Could you check a few things on this model? Use its own coordinates, in mm. Face numbers are marked on the shaded views. Round coordinates to 2 decimals unless told otherwise and drop trailing zeros. Order: outer loops, then holes, each group sorted by start corner. A loop starts at its lowest first (then second) coordinate and runs counter-clockwise, first axis right, second up.
```python
from build123d import *

# Parameters (mm, degrees)
EXTRUDE_1_DEPTH          = 30
SKETCH_2_R               = 3.5
CUT_EXTRUDE_1_DEPTH      = 71
SKETCH_3_R               = 3.5
CUT_EXTRUDE_2_DEPTH      = 71
SKETCH_4_R               = 4.5
SKETCH_4_R_2             = 2.5
EXTRUDE_2_DEPTH          = 30
SKETCH_5_R               = 2.5
CUT_EXTRUDE_6_DEPTH      = 31
SKETCH_6_W               = 11.97763243
SKETCH_6_H               = 9.98933257
CUT_EXTRUDE_8_DEPTH      = 71
CUT_EXTRUDE_8_DEPTH_BACK = 1.2


with BuildPart() as part:
    # Эскиз1 → Вытянуть-Тонкостенный1 (new body)
    with BuildSketch(Plane(origin=(0, 0, 0), x_dir=(1, 0, 0), z_dir=(0, 1, 0))):
        Polygon((0, 70), (0, 0), (70, 0), (70, 3), (3, 3), (3, 70), align=None)
    extrude(amount=EXTRUDE_1_DEPTH)

    # Эскиз2 → Вырез-Вытянуть1 (cut, through all)
    with BuildSketch(Plane.ZY):
        with Locations((-50, 20)):
            Circle(SKETCH_2_R)
        with Locations((-25, 10)):
            Circle(SKETCH_2_R)
    extrude(amount=-CUT_EXTRUDE_1_DEPTH, mode=Mode.SUBTRACT)

    # Эскиз3 → Вырез-Вытянуть2 (cut, through all)
    with BuildSketch(Plane.XY):
        with Locations((25, 20)):
            Circle(SKETCH_3_R)
        with Locations((50, 10)):
            Circle(SKETCH_3_R)
    extrude(amount=-CUT_EXTRUDE_2_DEPTH, mode=Mode.SUBTRACT)

    # Эскиз4 → Вытянуть-Тонкостенный2 (add)
    with BuildSketch(Plane(origin=(0, 0, 0), x_dir=(1, 0, 0), z_dir=(0, 1, 0))):
        with Locations((4.3, 71)):
            Circle(SKETCH_4_R)
        with Locations((4.3, 71)):
            Circle(SKETCH_4_R_2, mode=Mode.SUBTRACT)
    extrude(amount=EXTRUDE_2_DEPTH)

    # Эскиз5 → Вырез-Вытянуть6 (cut, through all)
    with BuildSketch(Plane(origin=(0, 0, 0), x_dir=(1, 0, 0), z_dir=(0, 1, 0))):
        with Locations((4.3, 71)):
            Circle(SKETCH_5_R)
    extrude(amount=CUT_EXTRUDE_6_DEPTH, mode=Mode.SUBTRACT)

    # Эскиз6 → Вырез-Вытянуть8 (cut, two sides)
    with BuildSketch(Plane(origin=(0, 0, 0), x_dir=(0, 0, -1), z_dir=(1, 0, 0))) as cut_extrude_8_sk:
        with Locations((70.813459228, 14.994666285)):
            Rectangle(SKETCH_6_W, SKETCH_6_H)
    extrude(amount=CUT_EXTRUDE_8_DEPTH, mode=Mode.SUBTRACT)
    extrude(cut_extrude_8_sk.sketch, amount=-CUT_EXTRUDE_8_DEPTH_BACK, mode=Mode.SUBTRACT)


solid = part.part
```
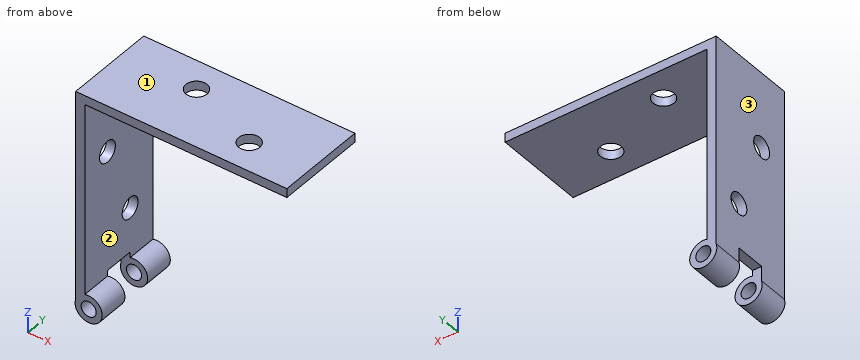
Q1. Imagine slicing it at C-C, the plane x = 50. Please give me the cut outline in (y, z), then the cut area to 3 significant figures.
Q2. Imagine slicing it at A-A, the plane y = 8.75. Please give me the cut outline in (x, z), then the cut area to 3 significant figures.
Q3. Imagine slicing it at B-B, the plane z = -25. Please give me the cut outline in (x, y).
Q4. We'd pull the mould along Z, two halves only. Please class the marked faces 1, 2 and 3: released by +Z, released by -Z, zero draft, split by the parting line, or undercut.
Q5. For P1, Ø1, axis at y = 20, z = -44, coming from the +X side; P2, Ø12, axis at x = 43, y = 22.5, coming from the +Z side; P3, Ø11, axis at y = 20, z = -50, coming from the -X side; P4, Ø1.5, axis at x = 2, y = 13, coming from the -Z side, each with a flat end and sliding along its axis, tell me the tip position at first contact or that it passes through.
Q6. Imagine slicing it at D-D, the plane y = 14.5. Please give me the cut outline in (x, z).
Q7. I need wall thicknesses on L1, parallel to Z at x = 4.3, y = 25.5; L2, parallel to Y at x = 0.6, z = -25; L3, parallel to Y at x = 25, z = -1. Which ranges of each line are inside material? Lowest first, please.
Filled in:
1. outline: (0, -3) - (6.5, -3) - (6.5, 0) - (0, 0) - close; (13.5, -3) - (30, -3) - (30, 0) - (13.5, 0) - close
1. area: 69.0 mm2
2. outline: (0, -69.67) arc R4.5 ccw (long way) to (3, -66.69) - (3, -28.27) - (0, -28.27) - close; (0, -21.73) - (3, -21.73) - (3, -3) - (46.73, -3) - (46.73, 0) - (0, 0) - close; (53.27, -3) - (70, -3) - (70, 0) - (53.27, 0) - close; hole circle Ø5 at (4.3, -71)
2. area: 409 mm2
3. outline: (0, 0) - (3, 0) - (3, 6.5) - (0, 6.5) - close; (0, 13.5) - (3, 13.5) - (3, 30) - (0, 30) - close
4. face 1: released by +Z
4. face 2: undercut
4. face 3: zero draft
5. P1: stops at x = 3
5. P2: stops at z = 0
5. P3: stops at x = 0
5. P4: stops at z = -64.82
6. outline: (0, -64.82) - (3, -64.82) - (3, -3) - (70, -3) - (70, 0) - (0, 0) - close
7. L1: z = -75.5 to -73.5, -68.5 to -66.5, -3 to 0
7. L2: y = 0 to 6.5, 13.5 to 30
7. L3: y = 0 to 16.5, 23.5 to 30
